```python
from build123d import *

# Parameters (mm, degrees)
PAD_DEPTH         = 100
SKETCH001_R       = 3
SKETCH001_R_2     = 1.6
POCKET_DEPTH      = 2.001
POCKET_DEPTH_BACK = 2.001
SKETCH004_R       = 11
SKETCH003_R       = 9
SKETCH005_R       = 11
FILLET_R          = 4
FILLET001_R       = 3


with BuildPart() as part:
    # Sketch → Pad (new body)
    with BuildSketch(Plane.YZ):
        Polygon((0, 2), (-20, 2), (-20, 0), (-20, -2), (0, -2), (20, -2), (20, 0), (20, 2), align=None)
    extrude(amount=PAD_DEPTH)

    # Sketch001 → Pocket (cut, two sides)
    with BuildSketch(Plane.XY) as pocket_sk:
        with Locations((30, 0)):
            Circle(SKETCH001_R)
        with Locations((4, 16)):
            Circle(SKETCH001_R_2)
        with Locations((4, -16)):
            Circle(SKETCH001_R_2)
        with Locations((96, 16)):
            Circle(SKETCH001_R_2)
        with Locations((96, -16)):
            Circle(SKETCH001_R_2)
    extrude(amount=-POCKET_DEPTH, mode=Mode.SUBTRACT)
    extrude(pocket_sk.sketch, amount=POCKET_DEPTH_BACK, mode=Mode.SUBTRACT)

    # Sketch004 (on DatumPlane) → SubtractiveLoft section 0
    with BuildSketch(Plane.XY.offset(2)):
        with Locations((63, 0)):
            Circle(SKETCH004_R)
    # Sketch003 → SubtractiveLoft section 1
    with BuildSketch(Plane.XY):
        with Locations((63, 0)):
            Circle(SKETCH003_R)
    # Sketch005 (on DatumPlane) → SubtractiveLoft section 2
    with BuildSketch(Plane.XY.offset(-2)):
        with Locations((63, 0)):
            Circle(SKETCH005_R)
    loft(ruled=True, mode=Mode.SUBTRACT)

    # Sketch007 (on DatumPlane) → SubtractiveLoft001 section 0
    with BuildSketch(Plane.XY.offset(2)):
        Polygon((63, 0), (63, 11), (113, 11), (113, -11), (63, -11), align=None)
    # Sketch006 → SubtractiveLoft001 section 1
    with BuildSketch(Plane.XY):
        Polygon((63, 0), (63, 9), (113, 9), (113, -9), (63, -9), align=None)
    # Sketch008 (on DatumPlane) → SubtractiveLoft001 section 2
    with BuildSketch(Plane.XY.offset(-2)):
        Polygon((63, 11), (63, 0), (63, -11), (113, -11), (113, 11), align=None)
    loft(ruled=True, mode=Mode.SUBTRACT)

    # Fillet
    fillet_edges = [part.edges().sort_by_distance(p)[0] for p in [
        (100, -20, 1),
        (100, 20, 1),
        (0, 20, 1),
        (0, -20, 1),
    ]]
    fillet(fillet_edges, radius=FILLET_R)

    # Fillet001
    fillet001_edges = [part.edges().sort_by_distance(p)[0] for p in [
        (100, -10, 1),
        (100, -10, -1),
        (100, 10, 1),
        (100, 10, -1),
    ]]
    fillet(fillet001_edges, radius=FILLET001_R)


solid = part.part
```
Model file for the job. Use its own axes, mm. A direction names the side the tool comes from. Give positions to 0.01 mm unless a question says otherwise; leave off trailing zeros. Loops run counter-clockwise (first coordinate to the right, second up) from the corner with the lowest first, then second, coordinate; pieces in that order, holes last. Notation, with made-up numbers: (0, -17) - (34, -17) arc R37 cw to (34, 21) - close; hole circle Ø1 at (63, -39.75). An arc over 180 degrees is marked (long way). One line per item, written item: value. Start each with the question number.
1. Probe L1, parallel to X at y = 16, z = 0.6; L2, parallel to Y at x = 4, z = 1.6; L3, parallel to Y at x = 59, z = 1.75. List the from-to ranges inside material, lowest first. Write a range as from..to.
2. Pin check, flat tips, straight feed: pin 1 (4 mm diameter, centred on x = 96, y = -16, fed in from +Z); pin 2 (1 mm diameter, centred on y = -13.5, z = -1.5, fed in from +X); pin 3 (1.5 mm diameter, centred on x = 64.5, y = 9.5, fed in from -Z). Stop position of each tip, or through.
3. Which spindle directions (+Z, -Z, +X, -X, +Y, -Y) get a long thin tool onto all of the face, cutting with end or side? Do faces 1 (the cylindrical face through (98.859, 18.797, 0.028)), 2 (the flat face through (80, 10, -1)), 3 (the cylindrical face through (99.145, 11.269, 0.994)). Say none if no direction does.
4. Slice it at A-A (x = 30). List the corners of the cut face in (y, z).
5. Slice it at B-B (z = 1.1). Give the number of separate pieces and of enclosed holes in the cut face, plus the area to 3 significant figures.
Solution:
1. L1: x = 0..2.4, 5.6..94.4, 97.6..100
1. L2: y = -20..-17.6, -14.4..14.4, 17.6..20
1. L3: y = -20..-9.98, 9.98..20
2. pin 1: stops at z = 2
2. pin 2: stops at x = 99.98
2. pin 3: stops at z = -1.25
3. face 1: +Z, -Z, +X, +Y
3. face 2: -Z, +X
3. face 3: +Z, +X
4. outline: (-20, -2) - (-3, -2) - (-3, 2) - (-20, 2) - close; (3, -2) - (20, -2) - (20, 2) - (3, 2) - close
5. separate pieces: 1
5. enclosed holes: 5
5. area: 3,010 mm^2
